from build123d import *

# Parameters (mm, degrees)
BOSS_EXTRUDE1_DEPTH = 56
SKETCH3_W           = 16
SKETCH3_H           = 36.624213763
CUT_EXTRUDE1_DEPTH  = 62.025698964
FILLET1_R           = 2


with BuildPart() as part:
    # Sketch2 → Boss-Extrude1 (new body)
    with BuildSketch(Plane.XY):
        with BuildLine():
            Line((-50.370168415, 15.39961681), (-55.370168415, 15.39961681))
            Line((-55.370168415, 15.39961681), (-55.370168415, 13.39961681))
            Line((-55.370168415, 13.39961681), (-50.370168415, 13.39961681))
            Line((-50.370168415, 13.39961681), (-50.370168415, 5.39961681))
            ThreePointArc((-50.370168415, 5.39961681), (-50.955954852, 3.985403248), (-52.370168415, 3.39961681))
            Line((-52.370168415, 3.39961681), (-57.370168415, 3.39961681))
            ThreePointArc((-57.370168415, 3.39961681), (-58.784381977, 2.813830372), (-59.370168415, 1.39961681))
            Line((-59.370168415, 1.39961681), (-59.370168415, -5.10038319))
            ThreePointArc((-59.370168415, -5.10038319), (-58.784381977, -6.514596752), (-57.370168415, -7.10038319))
            Line((-57.370168415, -7.10038319), (-52.370168415, -7.10038319))
            ThreePointArc((-52.370168415, -7.10038319), (-50.955954852, -7.686169628), (-50.370168415, -9.10038319))
            Line((-50.370168415, -9.10038319), (-50.370168415, -17.10038319))
            Line((-50.370168415, -17.10038319), (-43.370168415, -18.224596953))
            Line((-43.370168415, -18.224596953), (-43.370168415, -16.19896817))
            Line((-43.370168415, -16.19896817), (-48.370168415, -15.395958339))
            Line((-48.370168415, -15.395958339), (-48.370168415, -9.10038319))
            ThreePointArc((-48.370168415, -9.10038319), (-49.54174129, -6.271956065), (-52.370168415, -5.10038319))
            Line((-52.370168415, -5.10038319), (-57.370168415, -5.10038319))
            Line((-57.370168415, -5.10038319), (-57.370168415, 1.39961681))
            Line((-57.370168415, 1.39961681), (-52.370168415, 1.39961681))
            ThreePointArc((-52.370168415, 1.39961681), (-49.54174129, 2.571189685), (-48.370168415, 5.39961681))
            Line((-48.370168415, 5.39961681), (-48.370168415, 13.39961681))
            ThreePointArc((-48.370168415, 13.39961681), (-48.955954852, 14.813830372), (-50.370168415, 15.39961681))
        make_face()
    extrude(amount=BOSS_EXTRUDE1_DEPTH)

    # Sketch3 → Cut-Extrude1 (cut, through all)
    with BuildSketch(Plane.ZY.offset(59.370168415)):
        with Locations((28, -4.912490072)):
            Rectangle(SKETCH3_W, SKETCH3_H)
    extrude(amount=-CUT_EXTRUDE1_DEPTH, mode=Mode.SUBTRACT)

    # Fillet1
    fillet1_edges = [part.edges().sort_by_distance(p)[0] for p in [
        (-50.370168415, -17.10038319, 46),
        (-50.370168415, -17.10038319, 10),
    ]]
    fillet(fillet1_edges, radius=FILLET1_R)


solid = part.part
Verification items for the finished model (mm, model axes). A direction names the side the tool comes from. Give positions to 0.01 mm unless a question says otherwise; leave off trailing zeros. Write each loop counter-clockwise with the first axis right and the second up, starting at its lowest first coordinate (ties: lowest second). Pieces come first, ordered by that corner, then holes. Notation, with made-up numbers: (1.25, 24) - (34.25, 24) arc R32 cw to (34.25, 57) - close; hole circle Ø5 at (36, -34). An arc over 180 degrees is marked (long way). Answer as CSV lines item,"result". Start each with the question number.
1. Sectioned sample at B-B (y = 0). Record the boundary of the cut face in (x, z), then the cut area to 3 significant figures.
2. Thickness scan on line 1 (Z direction, x = -56.75, y = -5.5); line 2 (X direction, y = -4, z = 9); line 3 (Y direction, x = -53, z = 31). Record the ranges inside material, lowest first.
3. Draft check along Y on faces 5 (the face through (-50.37, -12, 46)), 6 (the face through (-48.94, 14.8, 27.61)), 7 (the face through (-57.37, -2, 10)). Enter one of: pulls with the +Y half, pulls with the -Y half, needs draft (parallel to the pull), parting line crosses it, or undercut.
4. Depth check by flat-ended pin: pin 1 (2 mm diameter, centred on x = -46.5, z = 37, fed in from -Y); pin 2 (12 mm diameter, centred on y = 6, z = 19.5, fed in from +X); pin 3 (4 mm diameter, centred on y = 8.5, z = 7, fed in from -X); pin 4 (2.5 mm diameter, centred on x = -56, z = 46, fed in from +Y). Enter the tip coordinate at first touch or a pass-through.
5. Sectioned sample at C-C (z = 10.5). Record the boundary of the cut face in (x, y), then the cut area to 3 significant figures.
6. Sectioned sample at A-A (x = -56.75). Record the boundary of the cut face in (y, z), then the cut area to 3 significant figures.
7. Sectioned sample at D-D (x = -47). Record the boundary of the cut face in (y, z).
8. Set-up check for faces 1 (the face through (-55, 1.4, 10)), 2 (the face through (-53, 13.4, 28)), 3 (the face through (-55.37, 14, 28)), 4 (the face through (-55, -7.1, 10)): record each of +Z, -Z, +X, -X, +Y, -Y from which the full face is reachable in a straight line by a thin tool's end or side.
Derived:
1,outline,"(-59.37, 0) - (-57.37, 0) - (-57.37, 20) - (-59.37, 20) - close; (-59.37, 36) - (-57.37, 36) - (-57.37, 56) - (-59.37, 56) - close"
1,area,"80.0 mm²"
2,line 1,"0 to 20, 36 to 56"
2,line 2,"-59.37 to -57.37"
2,line 3,"13.4 to 15.4"
3,face 5,"needs draft"
3,face 6,"pulls with the +Y half"
3,face 7,"undercut"
4,pin 1,"y = -17.88"
4,pin 2,"x = -48.37"
4,pin 3,"x = -50.37"
4,pin 4,"y = 15.4"
5,outline,"(-59.37, -5.1) arc R2 ccw to (-57.37, -7.1) - (-52.37, -7.1) arc R2 cw to (-50.37, -9.1) - (-50.37, -15.4) arc R2 ccw to (-48.69, -17.37) - (-43.37, -18.22) - (-43.37, -16.2) - (-48.37, -15.4) - (-48.37, -9.1) arc R4 ccw to (-52.37, -5.1) - (-57.37, -5.1) - (-57.37, 1.4) - (-52.37, 1.4) arc R4 ccw to (-48.37, 5.4) - (-48.37, 13.4) arc R2 ccw to (-50.37, 15.4) - (-55.37, 15.4) - (-55.37, 13.4) - (-50.37, 13.4) - (-50.37, 5.4) arc R2 cw to (-52.37, 3.4) - (-57.37, 3.4) arc R2 ccw to (-59.37, 1.4) - close"
5,area,"113 mm²"
6,outline,"(-7.1, 0) - (-5.1, 0) - (-5.1, 20) - (-7.1, 20) - close; (-7.1, 36) - (-5.1, 36) - (-5.1, 56) - (-7.1, 56) - close; (1.4, 0) - (3.4, 0) - (3.4, 20) - (1.4, 20) - close; (1.4, 36) - (3.4, 36) - (3.4, 56) - (1.4, 56) - close"
6,area,"160 mm²"
7,outline,"(-17.64, 0) - (-15.62, 0) - (-15.62, 20) - (-17.64, 20) - close; (-17.64, 36) - (-15.62, 36) - (-15.62, 56) - (-17.64, 56) - close"
8,face 1,"+Z, -Z, +X"
8,face 2,"-X"
8,face 3,"+Z, -Z, -X, +Y"
8,face 4,"+Z, -Z, -X, -Y"
